```python
from build123d import *

# Parameters (mm, degrees)
SKETCH1_W           = 101.6
SKETCH1_H           = 76.2
BOSS_EXTRUDE1_DEPTH = 2.54
SKETCH3_W           = 35.052
SKETCH3_H           = 56.134
SKETCH3_W_2         = 9.4
SKETCH3_H_2         = 11
BOSS_EXTRUDE4_DEPTH = 1.27
SKETCH2_W           = 12.065
SKETCH2_H           = 10.16
SKETCH2_W_2         = 81.28
SKETCH2_H_2         = 62.484
SKETCH2_H_3         = 12.065
SKETCH2_W_3         = 1.6
SKETCH2_H_4         = 0.8
BOSS_EXTRUDE5_DEPTH = 2.54
SKETCH2_3_R         = 0.508
CUT_EXTRUDE1_DEPTH  = 4.81


with BuildPart() as part:
    # Sketch1 → Boss-Extrude1 (new body)
    with BuildSketch(Plane(origin=(0, 0, 0), x_dir=(1, 0, 0), z_dir=(0, 1, 0))):
        Rectangle(SKETCH1_W, SKETCH1_H)
    extrude(amount=BOSS_EXTRUDE1_DEPTH)

    # Sketch3 → Boss-Extrude4 (add)
    with BuildSketch(Plane.XZ):
        with Locations((10.16, 10.033)):
            Rectangle(SKETCH3_W, SKETCH3_H)
        with Locations((-22.478, -32.6)):
            Rectangle(SKETCH3_W_2, SKETCH3_H_2)
    extrude(amount=BOSS_EXTRUDE4_DEPTH)

    # Sketch2 → Boss-Extrude5 (add)
    with BuildSketch(Plane(origin=(0, 2.54, 0), x_dir=(1, 0, 0), z_dir=(0, 1, 0))):
        with Locations((-33.9725, -31.496)):
            Rectangle(SKETCH2_W, SKETCH2_H)
        with Locations((-16.1925, -31.496)):
            Rectangle(SKETCH2_W, SKETCH2_H)
        with Locations((-6.096, 5.588)):
            Rectangle(SKETCH2_W_2, SKETCH2_H_2)
        with Locations((42.926, -19.6215)):
            Rectangle(SKETCH2_W, SKETCH2_H_3)
        with Locations((42.926, 28.8925)):
            Rectangle(SKETCH2_W, SKETCH2_H_3)
        with Locations((43.345, 1.302)):
            Rectangle(SKETCH2_W_3, SKETCH2_H_4)
        with Locations((43.345, 6.293)):
            Rectangle(SKETCH2_W_3, SKETCH2_H_4)
        with Locations((43.345, 11.284)):
            Rectangle(SKETCH2_W_3, SKETCH2_H_4)
    extrude(amount=BOSS_EXTRUDE5_DEPTH)

    # Sketch2_3 → Cut-Extrude1 (cut, through all)
    with BuildSketch(Plane(origin=(0, 2.54, 0), x_dir=(1, 0, 0), z_dir=(0, 1, 0))):
        with Locations((-48.26, -31.75)):
            Circle(SKETCH2_3_R)
        with Locations((38.1, -31.75)):
            Circle(SKETCH2_3_R)
        with Locations((38.1, 36.83)):
            Circle(SKETCH2_3_R)
    extrude(amount=-CUT_EXTRUDE1_DEPTH, mode=Mode.SUBTRACT)


solid = part.part
```
CAD build for the part. Positions are in the model's coordinates, mm. A direction names the side the tool comes from. Coordinates: 2 decimals unless noted, no trailing zeros. Loops run counter-clockwise (first coordinate to the right, second up) from the corner with the lowest first, then second, coordinate; pieces in that order, holes last. Notation, with made-up numbers: (40, 82.25) - (63, 82.25) arc R13 cw to (63, 87.25) - close; hole circle Ø9 at (88.5, -11.75). An arc over 180 degrees is marked (long way). Return JSON: item names as keys, results as strings.
1. 3-axis set-ups, long thin cutter, end or side, ignore diameter. For faces 1 (the flat face through (43, 4, 25.654)), 2 (the flat face through (-27.94, 4, 32)), 3 (the flat face through (48.958, 4, -29)), 4 (the flat face through (-7, 4, -36.83)), 5 (the flat face through (36.894, 4, 20)): which of +Z, -Z, +X, -X, +Y, -Y reach the whole face in a straight line?
Result:
{"face 1": "+Z, +X, -X, +Y", "face 2": "+Z, +Y", "face 3": "+Z, -Z, +X, +Y", "face 4": "-Z, +X, -X, +Y", "face 5": "+Z, -Z, +Y"}
2. Band-saw the part on A-A (y = 4). State how many separate pieces and enclosed holes the cut face has, and give its area (3 significant figures).
Result:
{"separate pieces": "8", "enclosed holes": "0", "area": "5,620 mm2"}
3. Band-saw the part on C-C (x = -13.5). Give the cut face in (y, z), and give its area (3 significant figures).
Result:
{"outline": "(0, -38.1) - (2.54, -38.1) - (2.54, -36.83) - (5.08, -36.83) - (5.08, 25.65) - (2.54, 25.65) - (2.54, 26.42) - (5.08, 26.42) - (5.08, 36.58) - (2.54, 36.58) - (2.54, 38.1) - (0, 38.1) - close", "area": "378 mm2"}
4. Band-saw the part on B-B (z = -14). Give the cut face in (x, y), and give its area (3 significant figures).
Result:
{"outline": "(-50.8, 0) - (-7.37, 0) - (-7.37, -1.27) - (27.69, -1.27) - (27.69, 0) - (50.8, 0) - (50.8, 2.54) - (34.54, 2.54) - (34.54, 5.08) - (-46.74, 5.08) - (-46.74, 2.54) - (-50.8, 2.54) - close", "area": "509 mm2"}
5. Band-saw the part on D-D (x = 6.5). Give the cut face in (y, z).
Result:
{"outline": "(-1.27, -18.03) - (0, -18.03) - (0, -38.1) - (2.54, -38.1) - (2.54, -36.83) - (5.08, -36.83) - (5.08, 25.65) - (2.54, 25.65) - (2.54, 38.1) - (-1.27, 38.1) - close"}
6. Mould opens along Z. For faces 6 (the flat face through (48.958, 4, 20)), 7 (the flat face through (-34, 4, 26.416)), 8 (the flat face through (-16, 4, 36.576)), 9 (the flat face through (43, 4, 13.589)) say: released by +Z, released by -Z, zero draft, split by the parting line, or undercut.
Result:
{"face 6": "zero draft", "face 7": "undercut", "face 8": "released by +Z", "face 9": "undercut"}
7. Drop flat-ended pins along their axis: pin 1 (1.3 mm diameter, centred on y = 4, z = -30.5, fed in from +X); pin 2 (0.6 mm diameter, centred on x = 11.5, y = -0.5, fed in from -Z); pin 3 (0.9 mm diameter, centred on y = 3.5, z = -6, fed in from +X) (3 decimals). Give the stop position or say it passes through.
Result:
{"pin 1": "stops at x = 48.96", "pin 2": "stops at z = -18.03", "pin 3": "stops at x = 44.145"}
8. Probe L1, parallel to X at y = 0.85, z = 31.75; L2, parallel to Z at x = 38.1, y = 1.75; L3, parallel to X at y = 3, z = -23. List the from-to ranges inside material, lowest first. Write a range as from..to.
Result:
{"L1": "x = -50.8..-48.77, -47.75..37.59, 38.61..50.8", "L2": "z = -38.1..-37.34, -36.32..31.24, 32.26..38.1", "L3": "x = -46.74..34.54, 36.89..48.96"}
